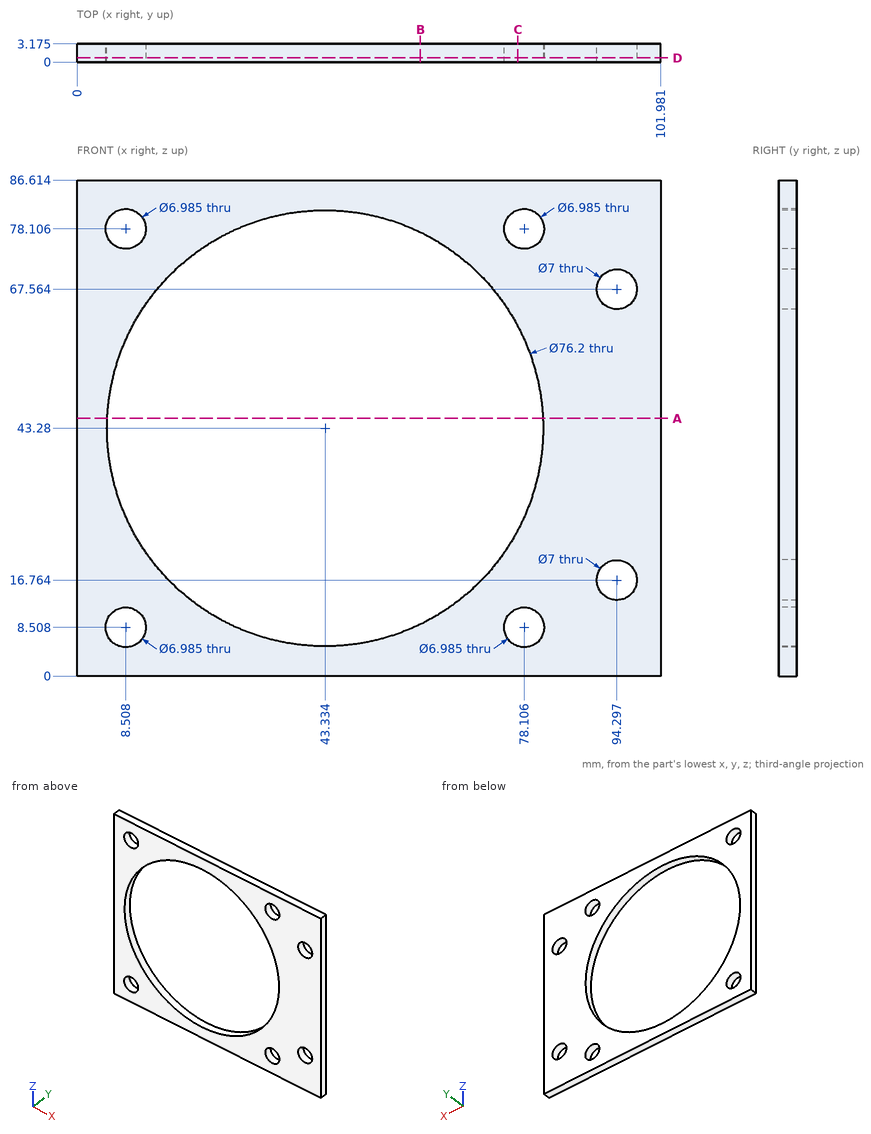
Job drawing, mm, ordinate dimensions from the low corner. One solid piece. Coordinates: 2 decimals unless noted, no trailing zeros. Order: outer loops, then holes, each group sorted by start corner. A loop starts at its lowest first (then second) coordinate and runs counter-clockwise, first axis right, second up. Notation, with made-up numbers: (-26, 9) -> (0, 9) arc R17 ccw to (0, 15) -> close; hole circle Ø4 at (89, 78). An arc over 180 degrees is marked (long way). Return JSON: item names as keys, results as strings. Group by question number.
Item 1: Saw through at D-D on y = 0.75. Write the cut outline in (x, z) (1 decimal).
Item 2: Saw through at C-C on x = 77. Write the cut outline in (y, z) (1 decimal).
Item 3: Saw through at B-B on x = 60. Write the cut outline in (y, z) (1 decimal).
Item 4: Saw through at A-A on z = 45. Write the cut outline in (x, y) (1 decimal).
Item 5: Wall check: line 1 along X through (y, z) = (2.85, 76.5) (1 decimal); line 2 along X through (y, z) = (0.45, 67.5) (1 decimal); line 3 along Z through (x, y) = (56.5, 2.75) (1 decimal). Give the ranges that are in metal, low to high. Write a range as [from, to].
Values found:
{
 "1": {"outline": "(0, 0) -> (102, 0) -> (102, 86.6) -> (0, 86.6) -> close; hole circle Ø7 at (8.5, 8.5); hole circle Ø7 at (8.5, 78.1); hole circle Ø76.2 at (43.3, 43.3); hole circle Ø7 at (78.1, 8.5); hole circle Ø7 at (78.1, 78.1); hole circle Ø7 at (94.3, 16.8); hole circle Ø7 at (94.3, 67.6)"},
 "2": {"outline": "(0, 0) -> (3.2, 0) -> (3.2, 5.2) -> (0, 5.2) -> close; (0, 11.8) -> (3.2, 11.8) -> (3.2, 25.4) -> (0, 25.4) -> close; (0, 61.1) -> (3.2, 61.1) -> (3.2, 74.8) -> (0, 74.8) -> close; (0, 81.4) -> (3.2, 81.4) -> (3.2, 86.6) -> (0, 86.6) -> close"},
 "3": {"outline": "(0, 0) -> (3.2, 0) -> (3.2, 9) -> (0, 9) -> close; (0, 77.5) -> (3.2, 77.5) -> (3.2, 86.6) -> (0, 86.6) -> close"},
 "4": {"outline": "(0, 0) -> (5.3, 0) -> (5.3, 3.2) -> (0, 3.2) -> close; (81.4, 0) -> (102, 0) -> (102, 3.2) -> (81.4, 3.2) -> close"},
 "5": {"line 1": "x = [0, 5.4], [11.6, 24.7], [62, 75], [81.2, 102]", "line 2": "x = [0, 13.9], [72.7, 90.8], [97.8, 102]", "line 3": "z = [0, 7.5], [79, 86.6]"}
}
